from build123d import *

# Parameters (mm, degrees)
SKETCH1_W           = 8.6
SKETCH1_H           = 4.4
BOSS_EXTRUDE1_DEPTH = 4.7
SKETCH4_W           = 4
SKETCH4_H           = 2
CUT_EXTRUDE1_DEPTH  = 0.9
SKETCH5_W           = 2
SKETCH5_H           = 2
BOSS_EXTRUDE3_DEPTH = 4.9
SKETCH7_W           = 0.4
SKETCH7_H           = 1.2
BOSS_EXTRUDE4_DEPTH = 2.8
CUT_EXTRUDE3_DEPTH  = 8.6
SKETCH9_W           = 0.5
SKETCH9_H           = 0.3
BOSS_EXTRUDE5_DEPTH = 2.8
FILLET1_R           = 0.25


with BuildPart() as part:
    # Sketch1 → Boss-Extrude1 (new body)
    with BuildSketch(Plane(origin=(0, 0, 0), x_dir=(1, 0, 0), z_dir=(0, 1, 0))):
        with Locations((4.3, -2.2)):
            Rectangle(SKETCH1_W, SKETCH1_H)
    extrude(amount=-BOSS_EXTRUDE1_DEPTH)

    # Sketch4 → Cut-Extrude1 (cut)
    with BuildSketch(Plane.XY.offset(4.4)):
        with Locations((4.3, -2.1)):
            Rectangle(SKETCH4_W, SKETCH4_H)
    extrude(amount=-CUT_EXTRUDE1_DEPTH, mode=Mode.SUBTRACT)

    # Sketch5 → Boss-Extrude3 (add)
    with BuildSketch(Plane.XY.offset(3.5)):
        with Locations((5.3, -2.1)):
            Rectangle(SKETCH5_W, SKETCH5_H)
    extrude(amount=BOSS_EXTRUDE3_DEPTH)

    # Sketch7 → Boss-Extrude4 (add)
    with BuildSketch(Plane.XZ.offset(4.7)):
        with Locations((0.2, 2.2)):
            Rectangle(SKETCH7_W, SKETCH7_H)
        with Locations((8.4, 2.2)):
            Rectangle(SKETCH7_W, SKETCH7_H)
    extrude(amount=BOSS_EXTRUDE4_DEPTH)

    # Sketch8 → Cut-Extrude3 (cut)
    with BuildSketch(Plane.ZY):
        with BuildLine():
            Line((1.9, -4.7), (1.6, -4.7))
            Line((1.6, -4.7), (1.6, -6.3))
            add(Edge.make_bspline(
                [(1.9, -4.7), (1.667864555, -5.492366311), (1.6, -6.3)],
                knots=[0, 0, 0, 0.547569636, 0.547569636, 0.547569636], degree=2))
        make_face()
        with BuildLine():
            add(Edge.make_bspline(
                [(2.5, -4.7), (2.732135445, -5.492366311), (2.8, -6.3)],
                knots=[0, 0, 0, 0.547569636, 0.547569636, 0.547569636], degree=2))
            Line((2.8, -6.3), (2.8, -4.7))
            Line((2.8, -4.7), (2.5, -4.7))
        make_face()
        with BuildLine():
            add(Edge.make_bspline(
                [(2.8, -6.3), (2.761794113, -6.997512334), (2.40000004, -7.5)],
                knots=[0, 0, 0, 0.682369162, 0.682369162, 0.682369162], degree=2))
            Line((2.40000004, -7.5), (2.8, -7.5))
            Line((2.8, -7.5), (2.8, -6.3))
        make_face()
        with BuildLine():
            add(Edge.make_bspline(
                [(1.6, -6.3), (1.638205887, -6.997512334), (1.99999996, -7.5)],
                knots=[0, 0, 0, 0.682369162, 0.682369162, 0.682369162], degree=2))
            Line((1.6, -6.3), (1.6, -7.5))
            Line((1.6, -7.5), (1.99999996, -7.5))
        make_face()
    extrude(amount=-CUT_EXTRUDE3_DEPTH, mode=Mode.SUBTRACT)

    # Sketch9 → Boss-Extrude5 (add)
    with BuildSketch(Plane.XZ.offset(4.7)):
        with Locations((4.3, 2.2)):
            Rectangle(SKETCH9_W, SKETCH9_H)
        with Locations((2.3, 2.2)):
            Rectangle(SKETCH9_W, SKETCH9_H)
        with Locations((6.3, 2.2)):
            Rectangle(SKETCH9_W, SKETCH9_H)
    extrude(amount=BOSS_EXTRUDE5_DEPTH)

    # Fillet1
    fillet1_edges = [part.edges().sort_by_distance(p)[0] for p in [
        (4.3, 0, 0),
        (8.6, 0, 2.2),
        (4.3, 0, 4.4),
        (0, 0, 2.2),
    ]]
    fillet(fillet1_edges, radius=FILLET1_R)


solid = part.part
Model file for the job. Use its own axes, mm. A direction names the side the tool comes from. Coordinates: 2 decimals unless noted, no trailing zeros. Write each loop counter-clockwise with the first axis right and the second up, starting at its lowest first coordinate (ties: lowest second). Pieces come first, ordered by that corner, then holes. Notation, with made-up numbers: (3, -24.5) -> (27, -24.5) arc R23 cw to (27, -12.5) -> close; hole circle Ø8 at (70, 2). An arc over 180 degrees is marked (long way). One line per item, written item: value. Start each with the question number.
1) Pull direction X, two halves, no side cores. Call faces 1 (the face through (3, -1.1, 4)), 2 (the face through (4, -2, 0)), 3 (the face through (2.3, -2, 4)), 4 (the face through (6.3, -2, 6)): +X half, -X half, draft (parallel to the pull), parting line (faces both ways), or undercut.
2) Slice it at C-C on z = 3. Write the cut outline in (x, y), then the cut area to 3 significant figures.
3) Slice it at D-D on y = -5.75. Count the separate pieces of the cut face and the enclosed holes in it, then the cut area to 3 significant figures.
4) Slice it at B-B on x = 5.75. Write the cut outline in (y, z).
5) Probe probe 1 along Y at (x, z) = (4.75, 2.5); probe 2 along Z at (x, y) = (1.5, -0.5); probe 3 along Z at (x, y) = (3.25, -2.75). List the from-to ranges inside material, lowest first.
6) Flat gauge pins, fed straight in: pin 1 Ø0.6 at (x, y) = (4.5, -5.5) entering from -Z; pin 2 Ø0.6 at (x, y) = (2.5, -6.5) entering from +Z; pin 3 Ø2 at (x, z) = (5, 6.5) entering from +Y; pin 4 Ø3.5 at (x, y) = (3.5, -3) entering from +Z. Where does each tip first touch, or does it go through?
7) Slice it at A-A on y = -1.5. Write the cut outline in (x, z), then the cut area to 3 significant figures.
8) Which spindle directions (+Z, -Z, +X, -X, +Y, -Y) get a long thin tool onto all of the face, cutting with end or side? Do faces 5 (the face through (8.2, -6, 2)), 6 (the face through (4.3, -2, 6)), 7 (the face through (5, -3.1, 6)), 8 (the face through (8.6, -3, 2)), 9 (the face through (5, -1.1, 6)). Say none if no direction does.
Answers follow:
1. face 1: undercut
1. face 2: draft
1. face 3: undercut
1. face 4: +X half
2. outline: (0, -4.7) -> (8.6, -4.7) -> (8.6, -0.25) arc R0.25 ccw to (8.35, 0) -> (0.25, 0) arc R0.25 ccw to (0, -0.25) -> close
2. area: 40.4 mm2
3. separate pieces: 5
3. enclosed holes: 0
3. area: 1.31 mm2
4. outline: (-4.7, 0) -> (-0.25, 0) arc R0.25 ccw to (0, 0.25) -> (0, 4.15) arc R0.25 ccw to (-0.25, 4.4) -> (-1.1, 4.4) -> (-1.1, 8.4) -> (-3.1, 8.4) -> (-3.1, 4.4) -> (-4.7, 4.4) -> close
5. probe 1: -4.7 to 0
5. probe 2: 0 to 4.4
5. probe 3: 0 to 3.5
6. pin 1: z = 2.05
6. pin 2: z = 2.35
6. pin 3: y = -1.1
6. pin 4: z = 8.4
7. outline: (0, 0) -> (8.6, 0) -> (8.6, 4.4) -> (6.3, 4.4) -> (6.3, 8.4) -> (4.3, 8.4) -> (4.3, 3.5) -> (2.3, 3.5) -> (2.3, 4.4) -> (0, 4.4) -> close
7. area: 44.0 mm2
8. face 5: +Z, -Z, -Y
8. face 6: +Z
8. face 7: +Z, +X, -X, -Y
8. face 8: +Z, -Z, +X, +Y, -Y
8. face 9: +Z, +X, -X, +Y
